Can you work these out from the drawing? Everything is in mm from the part's minimum corner. A direction names the side the tool comes from. Coordinates: 2 decimals unless noted, no trailing zeros. Write each loop counter-clockwise with the first axis right and the second up, starting at its lowest first coordinate (ties: lowest second). Pieces come first, ordered by that corner, then holes. Notation, with made-up numbers: (60.5, -7.75) -> (68.5, -7.75) arc R14 ccw to (68.5, 0.25) -> close; hole circle Ø10 at (-37, 87). An arc over 180 degrees is marked (long way). Use CSV: the item, a comma, the result in double quotes. Start each with the question number.
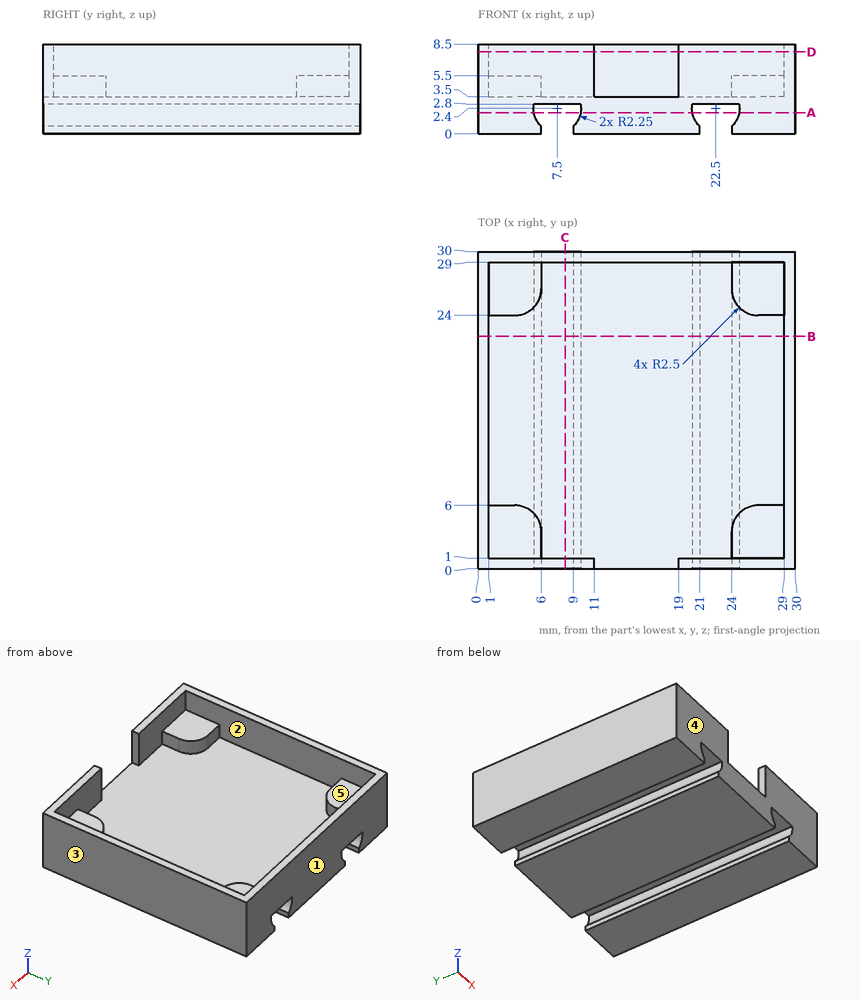
Item 1: Thinking about a two-plate mould opening in Y: for the marked faces 1, 2 and 3, which applies, +Y half, -Y half, draft (parallel to the pull), parting line (faces both ways), or undercut?
Item 2: I'm going to push flat-ended pins straight in: pin 1 (2 mm diameter, centred on x = 15.5, z = 6.5, fed in from -Y); pin 2 (6 mm diameter, centred on x = 8.5, y = 25.5, fed in from +Z); pin 3 (8 mm diameter, centred on x = 17, y = 21, fed in from +Z). Where does each tip first touch, or does it pass through?
Item 3: I want a section at A-A on z = 2. Please give me the cut outline in (x, y), then the cut area to 3 significant figures.
Item 4: I want a section at D-D on z = 7.75. Please give me the cut outline in (x, y), then the cut area to 3 significant figures.
Item 5: I want a section at B-B on y = 22. Please give me the cut outline in (x, z), then the cut area to 3 significant figures.
Item 6: I want a section at C-C on x = 8.25. Please give me the cut outline in (y, z), then the cut area to 3 significant figures.
Item 7: If I drill on line 1 along X through (y, z) = (6.25, 2.75); line 2 along X through (y, z) = (4, 0.5); line 3 along Y through (x, z) = (24.75, 7.5), over which ranges is the centre line in solid material (lowest first)?
Item 8: Which directions (+Z, -Z, +X, -X, +Y, -Y) give clear straight access to the entire face, cutting with the end or side of a thin tool? Please do the marked faces 4 and 5.
Geometry says:
1,face 1,"+Y half"
1,face 2,"undercut"
1,face 3,"draft"
2,pin 1,"y = 29"
2,pin 2,"z = 5.5"
2,pin 3,"z = 3.5"
3,outline,"(0, 0) -> (5.29, 0) -> (5.29, 30) -> (0, 30) -> close; (9.71, 0) -> (20.29, 0) -> (20.29, 30) -> (9.71, 30) -> close; (24.71, 0) -> (30, 0) -> (30, 30) -> (24.71, 30) -> close"
3,area,"634 mm2"
4,outline,"(0, 0) -> (11, 0) -> (11, 1) -> (1, 1) -> (1, 29) -> (29, 29) -> (29, 1) -> (19, 1) -> (19, 0) -> (30, 0) -> (30, 30) -> (0, 30) -> close"
4,area,"108 mm2"
5,outline,"(0, 0) -> (6, 0) -> (6, 0.72) arc R2.25 cw to (5.29, 2.8) -> (9.71, 2.8) arc R2.25 cw to (9, 0.72) -> (9, 0) -> (21, 0) -> (21, 0.72) arc R2.25 cw to (20.29, 2.8) -> (24.71, 2.8) arc R2.25 cw to (24, 0.72) -> (24, 0) -> (30, 0) -> (30, 8.5) -> (29, 8.5) -> (29, 3.5) -> (1, 3.5) -> (1, 8.5) -> (0, 8.5) -> close"
5,area,"93.5 mm2"
6,outline,"(0, 2.8) -> (30, 2.8) -> (30, 8.5) -> (29, 8.5) -> (29, 3.5) -> (1, 3.5) -> (1, 8.5) -> (0, 8.5) -> close"
6,area,"31.0 mm2"
7,line 1,"0 to 5.28, 9.72 to 20.28, 24.72 to 30"
7,line 2,"0 to 6, 9 to 21, 24 to 30"
7,line 3,"0 to 1, 29 to 30"
8,face 4,"+Z, -Z, +X, -X, -Y"
8,face 5,"+Z"
